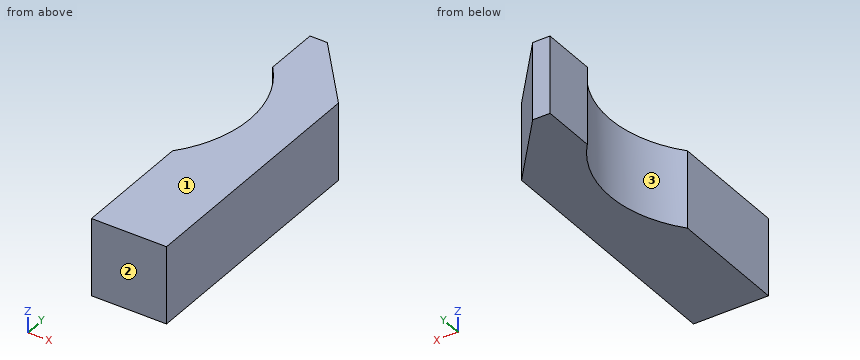
```python
from build123d import *

# Parameters (mm, degrees)
BOSS_EXTRUDE1_DEPTH = 33.02


with BuildPart() as part:
    # Sketch1 → Boss-Extrude1 (new body)
    with BuildSketch(Plane.XY):
        with BuildLine():
            Line((0, 0), (31.968493198, 0))
            Line((31.968493198, 0), (31.968493198, 109.242995925))
            Line((31.968493198, 109.242995925), (7.399294942, 138.771204316))
            Line((7.399294942, 138.771204316), (0, 138.771204316))
            Line((0, 138.771204316), (0, 115.1068086))
            ThreePointArc((0, 115.1068086), (11.60619963, 83.282987393), (0, 51.459166187))
            Line((0, 51.459166187), (0, 0))
        make_face()
    extrude(amount=BOSS_EXTRUDE1_DEPTH)


solid = part.part
```
Geometry check sheet. Reference: the model listing, model coordinates, mm. Face numbers are marked on the shaded views. Coordinates: 2 decimals unless noted, no trailing zeros. Order: outer loops, then holes, each group sorted by start corner. A loop starts at its lowest first (then second) coordinate and runs counter-clockwise, first axis right, second up.
Q1. Sectioned sample at C-C on y = 93.5. Record the cut outline in (x, z), and give its area (3 significant figures).
Reply:
outline: (10.54, 0) - (31.97, 0) - (31.97, 33.02) - (10.54, 33.02) - close
area: 708 mm2
Q2. Thickness scan on probe 1 along Y at (x, z) = (6, 13); probe 2 along Y at (x, z) = (3.5, 9); probe 3 along Y at (x, z) = (21, 21.5). Record the ranges inside material, lowest first.
Reply:
probe 1: y = 0 to 60.42, 106.15 to 138.77
probe 2: y = 0 to 56.16, 110.41 to 138.77
probe 3: y = 0 to 122.43
Q3. Depth check by flat-ended pin: pin 1 Ø6 at (x, y) = (20.5, 48) entering from -Z. Enter the tip coordinate at first touch or a pass-through.
Reply:
pin 1: stops at z = 0
Q4. Sectioned sample at B-B on z = 10.5. Record the cut outline in (x, y).
Reply:
outline: (0, 0) - (31.97, 0) - (31.97, 109.24) - (7.4, 138.77) - (0, 138.77) - (0, 115.11) arc R49.43 cw to (0, 51.46) - close
Q5. Sectioned sample at D-D on x = 23.5. Record the cut outline in (y, z).
Reply:
outline: (0, 0) - (119.42, 0) - (119.42, 33.02) - (0, 33.02) - close
Q6. Draft check along Y on the marked faces 1, 2 and 3. Enter one of: released by +Y, released by -Y, zero draft, split by the parting line, or undercut.
Reply:
face 1: zero draft
face 2: released by -Y
face 3: undercut
Q7. Sectioned sample at A-A on x = 9. Record the cut outline in (y, z), and give its area (3 significant figures).
Reply:
outline: (0, 0) - (67.44, 0) - (67.44, 33.02) - (0, 33.02) - close; (99.12, 0) - (136.85, 0) - (136.85, 33.02) - (99.12, 33.02) - close
area: 3,470 mm2
